Can you work these out from the model? Positions are in its coordinate system, mm. Face numbers are marked on the shaded views. Round coordinates to 2 decimals unless told otherwise and drop trailing zeros. Order: outer loops, then holes, each group sorted by start corner. A loop starts at its lowest first (then second) coordinate and runs counter-clockwise, first axis right, second up. Notation, with made-up numbers: (64.5, -6) -> (117.5, -6) arc R14 ccw to (117.5, 14) -> close; hole circle Ø8 at (61.25, -0.5). An arc over 180 degrees is marked (long way). Use a Markdown table: item, result. Add a question column.
Q1. I'm going to push flat-ended pins straight in: pin 1 Ø8 at (x, y) = (-15, 10.5) entering from +Z; pin 2 Ø10 at (x, z) = (22.5, -50) entering from +Y; pin 3 Ø1.7 at (x, y) = (-32.5, 15) entering from +Z; pin 4 Ø4 at (x, z) = (24, -4.5) entering from +Y. Where does each tip first touch, or does it pass through?
Q2. If we section it at D-D on z = -26: List the corners of the cut face in (x, y) for me, plus the area to 4 significant figures.
Q3. If we section it at A-A on z = 65: List the corners of the cut face in (x, y) for me, plus the area to 3 significant figures.
Q4. If we section it at B-B on y = 15: Give the number of separate pieces and of enclosed holes in the cut face, plus the area to 3 significant figures.
Q5. I need wall thicknesses on line 1 along X through (y, z) = (10.5, 60.5); line 2 along X through (y, z) = (1.7, -65); line 3 along Y through (x, z) = (-32, -70). Which ranges of each line are inside material? Lowest first, please. Write a range as [from, to].
Q6. We'd pull the mould along Z, two halves only. Please class the marked faces 1 and 2: +Z half, -Z half, draft (parallel to the pull), parting line (faces both ways), or undercut.
Q7. If we section it at C-C on x = -32.5: List the corners of the cut face in (y, z) for me, plus the area to 3 significant figures.
```python
from build123d import *

# Parameters (mm, degrees)
SKETCH1_W               = 70.5
SKETCH1_H               = 150
BOSS_EXTRUDE1_DEPTH     = 20
SKETCH2_R               = 1.4
CUT_EXTRUDE1_DEPTH      = 7
SKETCH3_W               = 59.5
SKETCH3_H               = 15
CUT_EXTRUDE2_DEPTH      = 156.378771072
CUT_EXTRUDE5_DEPTH      = 102.242283657
CUT_EXTRUDE5_DEPTH_BACK = 102.242283657
SKETCH7_W               = 110
SKETCH7_H               = 15
FILLET1_R               = 5
SKETCH5_R               = 1.4
CUT_EXTRUDE3_DEPTH      = 85.217352725
CUT_EXTRUDE4_DEPTH      = 85.217352725
LPATTERN1_COUNT         = 5
LPATTERN1_PITCH         = 13
LPATTERN1_COL_COUNT     = 5
LPATTERN1_COL_PITCH     = 13


with BuildPart() as part:
    # Sketch1 → Boss-Extrude1 (new body)
    with BuildSketch(Plane(origin=(0, 0, 0), x_dir=(1, 0, 0), z_dir=(0, 1, 0))):
        Rectangle(SKETCH1_W, SKETCH1_H)
    extrude(amount=BOSS_EXTRUDE1_DEPTH)

    # Sketch2 → Cut-Extrude1 (cut)
    with BuildSketch(Plane(origin=(0, 0, -75), x_dir=(-1, 0, 0), z_dir=(0, 0, -1))):
        with Locations((-32.5, 15)):
            Circle(SKETCH2_R)
        with Locations(Location((-32.5, 5, 0), (0, 0, 180))):
            Circle(SKETCH2_R)
        with Locations((32.5, 5)):
            Circle(SKETCH2_R)
        with Locations(Location((32.5, 15, 0), (0, 0, 180))):
            Circle(SKETCH2_R)
    cut_extrude1 = extrude(amount=-CUT_EXTRUDE1_DEPTH, mode=Mode.SUBTRACT)

    # Sketch3 → Cut-Extrude2 (cut, through all)
    with BuildSketch(Plane.XY.offset(75)):
        with Locations((0, 12.5)):
            Rectangle(SKETCH3_W, SKETCH3_H)
    extrude(amount=-CUT_EXTRUDE2_DEPTH, mode=Mode.SUBTRACT)

    # Sketch7 → Cut-Extrude5 (cut, two sides: drawn at the far end of the back side and taken through both)
    with BuildSketch(Plane.ZY.offset(-29.75).offset(-CUT_EXTRUDE5_DEPTH_BACK)):
        with Locations((0, 12.5)):
            Rectangle(SKETCH7_W, SKETCH7_H)
    extrude(amount=CUT_EXTRUDE5_DEPTH + CUT_EXTRUDE5_DEPTH_BACK, mode=Mode.SUBTRACT)

    # Fillet1
    fillet1_edges = [part.edges().sort_by_distance(p)[0] for p in [
        (-29.75, 5, -65),
        (29.75, 5, -65),
        (29.75, 5, 65),
        (-29.75, 5, 65),
        (-32.5, 5, 55),
        (32.5, 5, 55),
        (-32.5, 5, -55),
        (32.5, 5, -55),
    ]]
    fillet(fillet1_edges, radius=FILLET1_R)

    # Sketch5 → Cut-Extrude3 (cut, through all)
    with BuildSketch(Plane(origin=(0, 5, 0), x_dir=(1, 0, 0), z_dir=(0, 1, 0))):
        with Locations(Location((-2.5, -70, 0), (0, 0, 270))):
            Circle(SKETCH5_R)
        with Locations(Location((2.5, -70, 0), (0, 0, 90))):
            Circle(SKETCH5_R)
        with Locations(Location((2.5, -65, 0), (0, 0, 270))):
            Circle(SKETCH5_R)
        with Locations(Location((-2.5, -65, 0), (0, 0, 90))):
            Circle(SKETCH5_R)
    cut_extrude3 = extrude(amount=-CUT_EXTRUDE3_DEPTH, mode=Mode.SUBTRACT)

    # Mirror1: Cut-Extrude1, Cut-Extrude3 across plane
    add(cut_extrude1.mirror(Plane.XY), mode=Mode.SUBTRACT)
    add(cut_extrude3.mirror(Plane.XY), mode=Mode.SUBTRACT)

    # Sketch6 → Cut-Extrude4 (cut, through all)
    with BuildSketch(Plane(origin=(0, 5, 0), x_dir=(1, 0, 0), z_dir=(0, 1, 0))):
        with BuildLine():
            Line((-17.5, 4), (17.5, 4))
            ThreePointArc((17.5, 4), (21.5, 0), (17.5, -4))
            Line((17.5, -4), (-17.5, -4))
            ThreePointArc((-17.5, -4), (-21.5, 0), (-17.5, 4))
        make_face()
    cut_extrude4 = extrude(amount=-CUT_EXTRUDE4_DEPTH, mode=Mode.SUBTRACT)

    # LPattern1: Cut-Extrude4 ×5
    with Locations(*[(0, 0, i * LPATTERN1_PITCH) for i in range(1, LPATTERN1_COUNT)]):
        add(cut_extrude4, mode=Mode.SUBTRACT)

    # LPattern1 col: Cut-Extrude4 ×5
    with Locations(*[(0, 0, -i * LPATTERN1_COL_PITCH) for i in range(1, LPATTERN1_COL_COUNT)]):
        add(cut_extrude4, mode=Mode.SUBTRACT)


solid = part.part
```
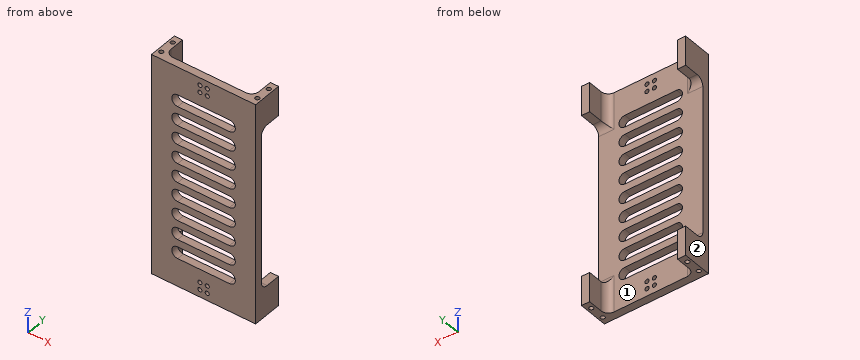
Answer below:
| question | item | result |
|---|---|---|
| 1 | pin 1 | through |
| 1 | pin 2 | y = 5.52 |
| 1 | pin 3 | z = 68 |
| 1 | pin 4 | y = 5 |
| 2 | outline | (-35.25, 0) -> (-21.5, 0) -> (-21.5, 5) -> (-35.25, 5) -> close; (21.5, 0) -> (35.25, 0) -> (35.25, 5) -> (21.5, 5) -> close |
| 2 | area | 137.5 mm² |
| 3 | outline | (-35.25, 0) -> (-3.9, 0) -> (-3.9, 5) -> (-24.75, 5) arc R5 cw to (-29.75, 10) -> (-29.75, 20) -> (-35.25, 20) -> close; (-1.1, 0) -> (1.1, 0) -> (1.1, 5) -> (-1.1, 5) -> close; (3.9, 0) -> (35.25, 0) -> (35.25, 20) -> (29.75, 20) -> (29.75, 10) arc R5 cw to (24.75, 5) -> (3.9, 5) -> close |
| 3 | area | 500 mm² |
| 4 | separate pieces | 4 |
| 4 | enclosed holes | 0 |
| 4 | area | 362 mm² |
| 5 | line 1 | [-35.25, -29.75], [29.75, 35.25] |
| 5 | line 2 | [-35.25, -3.9], [-1.1, 1.1], [3.9, 35.25] |
| 5 | line 3 | [0, 3.69], [6.31, 13.69], [16.31, 20] |
| 6 | face 1 | undercut |
| 6 | face 2 | draft |
| 7 | outline | (0, -75) -> (3.6, -75) -> (3.6, -68) -> (6.4, -68) -> (6.4, -75) -> (13.6, -75) -> (13.6, -68) -> (16.4, -68) -> (16.4, -75) -> (20, -75) -> (20, -55) -> (10, -55) arc R5 cw to (5, -50) -> (5, 50) arc R5 cw to (10, 55) -> (20, 55) -> (20, 75) -> (16.4, 75) -> (16.4, 68) -> (13.6, 68) -> (13.6, 75) -> (6.4, 75) -> (6.4, 68) -> (3.6, 68) -> (3.6, 75) -> (0, 75) -> close |
| 7 | area | 1,280 mm² |
